Check sheet for the modelled part. Datum: model origin and axes. Units: mm. Face numbers are marked on the shaded views. A direction names the side the tool comes from. Give positions to 0.01 mm unless a question says otherwise; leave off trailing zeros. Order: outer loops, then holes, each group sorted by start corner. A loop starts at its lowest first (then second) coordinate and runs counter-clockwise, first axis right, second up.
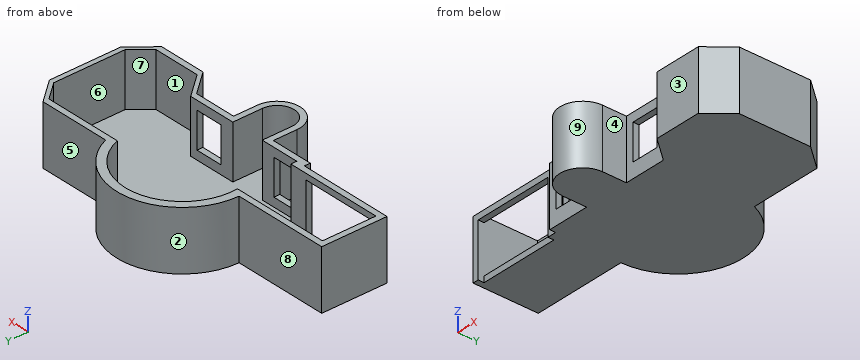
```python
from build123d import *

# Parameters (mm, degrees)
F1_DEPTH = 254
F3_DEPTH = 228.6
F5_W     = 118.080845
F5_H     = 152.4
F4_W     = 342.9
F4_H     = 228.6
F6_DEPTH = 25.4


with BuildPart() as f1:
    # F0 (on Top) → F1 (new body)
    with BuildSketch(Plane.XY):
        with BuildLine():
            Line((97.819155, -152.4), (279.4, -152.4))
            Line((279.4, -152.4), (364.652523, -254))
            Line((364.652523, -254), (567.852523, -254))
            Line((567.852523, -254), (653.105045, -152.4))
            Line((653.105045, -152.4), (653.105045, 152.4))
            Line((653.105045, 152.4), (567.852523, 254))
            Line((567.852523, 254), (260.272549, 254))
            ThreePointArc((260.272549, 254), (-51.692406, 426.976501), (-279.4, 152.4))
            Line((-279.4, 152.4), (-685.8, 152.4))
            Line((-685.8, 152.4), (-685.8, -127))
            Line((-685.8, -127), (-279.4, -127))
            Line((-279.4, -127), (-279.4, -152.4))
            Line((-279.4, -152.4), (-97.819155, -152.4))
            Line((-97.819155, -152.4), (-97.819155, -254))
            ThreePointArc((-97.819155, -254), (0, -351.819155), (97.819155, -254))
            Line((97.819155, -254), (97.819155, -152.4))
        make_face()
    extrude(amount=F1_DEPTH)

    # F2 (on face) → F3 (cut)
    with BuildSketch(Plane.XY.offset(254)):
        with BuildLine():
            Line((72.419155, -127), (242.20781, -127))
            Line((242.20781, -127), (279.4, -127))
            Line((279.4, -127), (364.652523, -228.6))
            Line((364.652523, -228.6), (567.852523, -228.6))
            Line((567.852523, -228.6), (631.791914, -152.4))
            Line((631.791914, -152.4), (631.791914, 152.4))
            Line((631.791914, 152.4), (567.852523, 228.6))
            Line((567.852523, 228.6), (231.307897, 228.6))
            ThreePointArc((231.307897, 228.6), (-51.091506, 390.516445), (-242.20781, 127))
            Line((-242.20781, 127), (-660.4, 127))
            Line((-660.4, 127), (-660.4, -101.6))
            Line((-660.4, -101.6), (-242.20781, -101.6))
            Line((-242.20781, -101.6), (-242.20781, -127))
            Line((-242.20781, -127), (-72.419155, -127))
            Line((-72.419155, -127), (-72.419155, -254))
            ThreePointArc((-72.419155, -254), (0, -326.419155), (72.419155, -254))
            Line((72.419155, -254), (72.419155, -127))
        make_face()
    extrude(amount=-F3_DEPTH, mode=Mode.SUBTRACT)

    # F5 (on face) + F4 (on face) → F6 (cut)
    with BuildSketch(Plane.XZ.offset(152.4)):
        with Locations((-188.609578, 139.7)):
            Rectangle(F5_W, F5_H)
        with Locations((189.446623, 139.7)):
            Rectangle(F5_W, F5_H)
    with BuildSketch(Plane.XZ.offset(127)):
        with Locations((-488.95, 114.3)):
            Rectangle(F4_W, F4_H)
    extrude(amount=-F6_DEPTH, mode=Mode.SUBTRACT)


solid = f1.part
```
(1) Cross-section at C-C on z = 162. Count the separate pieces of the cut face and the enclosed holes in it, then the cut area to 3 significant figures.
Response values:
separate pieces: 3
enclosed holes: 0
area: 88,100 mm2
(2) Gauge pin test, flat ends, axial feed: pin 1 Ø10 at (x, z) = (370, 157.5) entering from -Y; pin 2 Ø12 at (x, y) = (-330.5, 142.5) entering from -Z; pin 3 Ø1.5 at (y, z) = (-165.5, 171.5) entering from +X; pin 4 Ø12 at (y, z) = (313.5, 125) entering from -X. Record the tip position at first contact, or that the pin passes through.
Response values:
pin 1: stops at y = -254
pin 2: stops at z = 0
pin 3: stops at x = 642.74
pin 4: stops at x = -232.4
(3) Cross-section at A-A on x = 146.5. Enter the section's corners in (y, z), then the cut area to 3 significant figures.
Response values:
outline: (-152.4, 0) - (390.31, 0) - (390.31, 254) - (346.94, 254) - (346.94, 25.4) - (-127, 25.4) - (-127, 63.5) - (-152.4, 63.5) - close; (-152.4, 215.9) - (-127, 215.9) - (-127, 254) - (-152.4, 254) - close
area: 25,600 mm2
(4) Cross-section at B-B on y = 15. Enter the section's corners in (x, z), then the cut area to 3 significant figures.
Response values:
outline: (-685.8, 0) - (653.11, 0) - (653.11, 254) - (631.79, 254) - (631.79, 25.4) - (-660.4, 25.4) - (-660.4, 254) - (-685.8, 254) - close
area: 44,700 mm2
(5) Material ranges on L1, parallel to X at y = 95, z = 192.5; L2, parallel to Y at x = 562, z = 204.5; L3, parallel to X at y = -118, z = 151.5, recorded low to high.
Response values:
L1: x = -685.8 to -660.4, 631.79 to 653.11
L2: y = -254 to -228.6, 228.6 to 254
L3: x = -685.8 to -660.4, -317.5 to -242.21, 631.79 to 653.11
(6) Cross-section at D-D on x = 0. Enter the section's corners in (y, z), then the cut area to 3 significant figures.
Response values:
outline: (-351.82, 0) - (431.8, 0) - (431.8, 254) - (395.94, 254) - (395.94, 25.4) - (-326.42, 25.4) - (-326.42, 254) - (-351.82, 254) - close
area: 33,900 mm2
(7) Release check for a two-part mould opening along Y. For the marked faces 6, 7, 8 and 9 record: released by +Y, released by -Y, zero draft, split by the parting line, or undercut.
Response values:
face 6: undercut
face 7: undercut
face 8: released by +Y
face 9: released by -Y
(8) Set-up check for the marked faces 1, 2, 3, 4 and 5: record each of +Z, -Z, +X, -X, +Y, -Y from which the full face is reachable in a straight line by a thin tool's end or side.
Response values:
face 1: +Z
face 2: +Z, -Z, +Y
face 3: +Z, -Z, +X, -Y
face 4: +Z, -Z, -Y
face 5: +Z, -Z, +X, +Y
